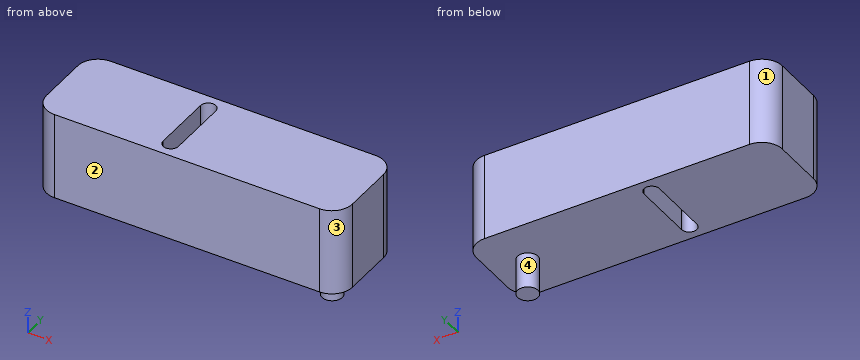
from build123d import *

# Parameters (mm, degrees)
SKETCH1_W           = 76.2
SKETCH1_H           = 22.86
BOSS_EXTRUDE1_DEPTH = 21.717
CUT_EXTRUDE3_REACH  = 23.717
FILLET1_R           = 5.08
SKETCH3_R           = 2.54
BOSS_EXTRUDE2_DEPTH = 8.89


with BuildPart() as part:
    # Sketch1 → Boss-Extrude1 (new body)
    with BuildSketch(Plane.XY):
        Rectangle(SKETCH1_W, SKETCH1_H)
    extrude(amount=-BOSS_EXTRUDE1_DEPTH)

    # Sketch2 → Cut-Extrude3 (cut, up to next)
    with BuildSketch(Plane.XY, mode=Mode.PRIVATE) as cut_extrude3_sk1:
        with BuildLine():
            Line((-8.255, -7.62), (-8.255, 7.62))
            ThreePointArc((-8.255, 7.62), (-6.35, 9.525), (-4.445, 7.62))
            Line((-4.445, 7.62), (-4.445, -7.62))
            ThreePointArc((-4.445, -7.62), (-6.35, -9.525), (-8.255, -7.62))
        make_face()
    cut_extrude3_tool1 = extrude(cut_extrude3_sk1.sketch, amount=-CUT_EXTRUDE3_REACH, mode=Mode.PRIVATE) & part.part
    add(cut_extrude3_tool1.solids().sort_by_distance((-6.35, 0, 0))[0], mode=Mode.SUBTRACT)

    # Fillet1
    fillet1_edges = [part.edges().sort_by_distance(p)[0] for p in [
        (38.1, -11.43, -10.8585),
        (-38.1, -11.43, -10.8585),
        (-38.1, 11.43, -10.8585),
        (38.1, 11.43, -10.8585),
    ]]
    fillet(fillet1_edges, radius=FILLET1_R)

    # Sketch3 → Boss-Extrude2 (add)
    with BuildSketch(Plane(origin=(0, 0, -21.717), x_dir=(-1, 0, 0), z_dir=(0, 0, -1))):
        with Locations((-29.21, 0)):
            Circle(SKETCH3_R)
    extrude(amount=BOSS_EXTRUDE2_DEPTH)


solid = part.part
Design review of the part built by this model. Coordinates are the model's own, in mm. Face numbers are marked on the shaded views. Coordinates: 2 decimals unless noted, no trailing zeros. Order: outer loops, then holes, each group sorted by start corner. A loop starts at its lowest first (then second) coordinate and runs counter-clockwise, first axis right, second up. Notation, with made-up numbers: (-28, 56.25) -> (23, 56.25) arc R23 ccw to (23, 73.25) -> close; hole circle Ø3 at (8.25, -39). An arc over 180 degrees is marked (long way). Use one line per item in the form item = value. Start each with the question number.
(1) Add section D-D on z = -25. State the section outline as (x, y) points, plus the area to 3 significant figures.
(2) The part is to be moulded in two halves that separate along X. For the marked faces 1, 2, 3 and 4, say which applies: +X half, -X half, draft (parallel to the pull), parting line (faces both ways), or undercut.
(3) Insertion check: pin 1 (10 mm diameter, centred on x = 22, z = -25.5, fed in from +Y); pin 2 (6 mm diameter, centred on x = 0.5, y = 6, fed in from -Z); pin 3 (4 mm diameter, centred on y = -9, z = -15.5, fed in from +X). Each pin has a flat end and moves straight along its axis. Give the tip position at first contact, or say it passes through.
(4) Add section C-C on z = -6.5. State the section outline as (x, y) points (3 decimals).
(5) Add section A-A on x = 29.21. State the section outline as (y, z) points, plus the area to 3 significant figures.
(6) Add section B-B on y = 0. State the section outline as (x, z) points (3 decimals), plus the area to 3 significant figures.
(7) For probe 1 along X at (y, z) = (-4.75, -8.5) (3 decimals); probe 2 along Z at (x, y) = (-13.5, -2); probe 3 along X at (y, z) = (9, -9.5), list the stretches that pass through material, from the lowest coordinate up.
Answer block:
q1.outline = circle Ø5.08 at (29.21, 0)
q1.area = 20.3 mm²
q2.face_1 = -X half
q2.face_2 = draft
q2.face_3 = +X half
q2.face_4 = parting line
q3.pin_1 = 11.43
q3.pin_2 = -21.72
q3.pin_3 = 38.06
q4.outline = (-38.1, -6.35) arc R5.08 ccw to (-33.02, -11.43) -> (33.02, -11.43) arc R5.08 ccw to (38.1, -6.35) -> (38.1, 6.35) arc R5.08 ccw to (33.02, 11.43) -> (-33.02, 11.43) arc R5.08 ccw to (-38.1, 6.35) -> close; hole (-8.255, -7.62) arc R1.905 ccw to (-4.445, -7.62) -> (-4.445, 7.62) arc R1.905 ccw to (-8.255, 7.62) -> close
q5.outline = (-11.43, -21.72) -> (-2.54, -21.72) -> (-2.54, -30.61) -> (2.54, -30.61) -> (2.54, -21.72) -> (11.43, -21.72) -> (11.43, 0) -> (-11.43, 0) -> close
q5.area = 542 mm²
q6.outline = (-38.1, -21.717) -> (-8.255, -21.717) -> (-8.255, 0) -> (-38.1, 0) -> close; (-4.445, -21.717) -> (26.67, -21.717) -> (26.67, -30.607) -> (31.75, -30.607) -> (31.75, -21.717) -> (38.1, -21.717) -> (38.1, 0) -> (-4.445, 0) -> close
q6.area = 1,620 mm²
q7.probe_1 = -38.1 to -8.255, -4.445 to 38.1
q7.probe_2 = -21.72 to 0
q7.probe_3 = -37.35 to -7.66, -5.04 to 37.35
